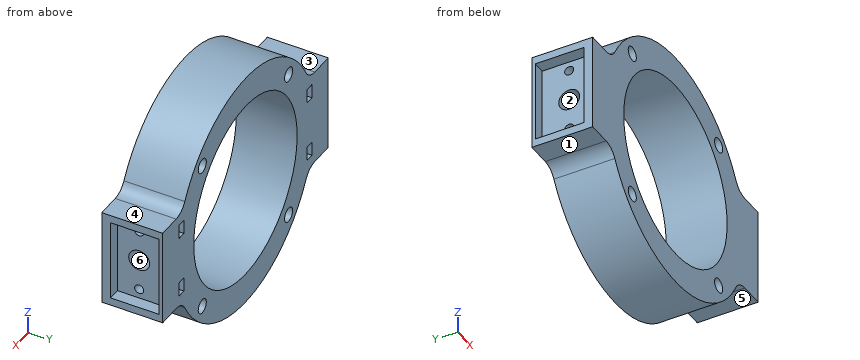
```python
from build123d import *

# Parameters (mm, degrees)
IZIM1_R                     = 52.5
Y_KSEKLIK_EKSTR_ZYON1_DEPTH = 35
IZIM2_R                     = 6.01
KES_EKSTR_ZYON1_DEPTH       = 27.24
IZIM3_W                     = 47
IZIM3_H                     = 28
KES_EKSTR_ZYON2_DEPTH       = 7
IZIM4_R                     = 2.6
KES_EKSTR_ZYON3_DEPTH       = 20
KES_EKSTR_ZYON4_DEPTH       = 2.45
IZIM7_R                     = 4.1
KES_EKSTR_ZYON5_DEPTH       = 115.808536268
RADYUS1_R                   = 10


with BuildPart() as part:
    # Çizim1 → Yükseklik-Ekstrüzyon1 (new body)
    with BuildSketch(Plane(origin=(0, 0, 0), x_dir=(1, 0, 0), z_dir=(0, 1, 0))):
        with BuildLine():
            Line((-64.156059729, 28), (-84, 28))
            Line((-84, 28), (-84, -28))
            Line((-84, -28), (-64.156059729, -28))
            ThreePointArc((-64.156059729, -28), (0, -70), (64.156059729, -28))
            Line((64.156059729, -28), (84, -28))
            Line((84, -28), (84, 28))
            Line((84, 28), (64.156059729, 28))
            ThreePointArc((64.156059729, 28), (0, 70), (-64.156059729, 28))
        make_face()
        with Locations(Location((0, 0, 0), (0, 0, 270))):
            Circle(IZIM1_R, mode=Mode.SUBTRACT)
    extrude(amount=Y_KSEKLIK_EKSTR_ZYON1_DEPTH)

    # Çizim2 → Kes-Ekstrüzyon1 (cut)
    with BuildSketch(Plane(origin=(84, 0, 0), x_dir=(0, 0, -1), z_dir=(1, 0, 0))):
        with Locations((0, 17.5)):
            Circle(IZIM2_R)
    kes_ekstr_zyon1 = extrude(amount=-KES_EKSTR_ZYON1_DEPTH, mode=Mode.SUBTRACT)

    # Aynalama1: Kes-Ekstrüzyon1 across plane
    add(kes_ekstr_zyon1.mirror(Plane(origin=(0, 0, 0), x_dir=(0, 0, 1), z_dir=(1, 0, 0))), mode=Mode.SUBTRACT)

    # Çizim3 → Kes-Ekstrüzyon2 (cut)
    with BuildSketch(Plane(origin=(84, 0, 0), x_dir=(0, 0, -1), z_dir=(1, 0, 0))):
        with Locations((0, 19)):
            Rectangle(IZIM3_W, IZIM3_H)
    kes_ekstr_zyon2 = extrude(amount=-KES_EKSTR_ZYON2_DEPTH, mode=Mode.SUBTRACT)

    # Aynalama2: Kes-Ekstrüzyon2 across plane
    add(kes_ekstr_zyon2.mirror(Plane(origin=(0, 0, 0), x_dir=(0, 0, 1), z_dir=(1, 0, 0))), mode=Mode.SUBTRACT)

    # Çizim4 → Kes-Ekstrüzyon3 (cut)
    with BuildSketch(Plane(origin=(77, 0, 0), x_dir=(0, 0, -1), z_dir=(1, 0, 0))):
        with Locations((18, 17.5)):
            Circle(IZIM4_R)
        with Locations(Location((-18, 17.5, 0), (0, 0, 180))):
            Circle(IZIM4_R)
    kes_ekstr_zyon3 = extrude(amount=-KES_EKSTR_ZYON3_DEPTH, mode=Mode.SUBTRACT)

    # Aynalama3: Kes-Ekstrüzyon3 across plane
    add(kes_ekstr_zyon3.mirror(Plane(origin=(0, 0, 0), x_dir=(0, 0, 1), z_dir=(1, 0, 0))), mode=Mode.SUBTRACT)

    # Çizim6 → Kes-Ekstrüzyon4 (cut, symmetric)
    with BuildSketch(Plane.ZY.offset(65)):
        Polygon((-22.1, 35), (-13.9, 35), (-13.9, 15.132863896), (-18, 12.765727793), (-22.1, 15.132863896), align=None)
        Polygon((18, 12.765727793), (22.1, 15.132863896), (22.1, 35), (13.9, 35), (13.9, 15.132863896), align=None)
    kes_ekstr_zyon4 = extrude(amount=KES_EKSTR_ZYON4_DEPTH, both=True, mode=Mode.SUBTRACT)

    # Aynalama4: Kes-Ekstrüzyon4 across plane
    add(kes_ekstr_zyon4.mirror(Plane(origin=(0, 0, 0), x_dir=(0, 0, 1), z_dir=(1, 0, 0))), mode=Mode.SUBTRACT)

    # Çizim7 → Kes-Ekstrüzyon5 (cut, through all)
    with BuildSketch(Plane(origin=(0, 35, 0), x_dir=(1, 0, 0), z_dir=(0, 1, 0))):
        with Locations(Location((43.840620434, -43.840620434, 0), (0, 0, 270))):
            Circle(IZIM7_R)
        with Locations(Location((-43.840620434, -43.840620434, 0), (0, 0, 270))):
            Circle(IZIM7_R)
        with Locations(Location((-43.840620434, 43.840620434, 0), (0, 0, 270))):
            Circle(IZIM7_R)
        with Locations(Location((43.840620434, 43.840620434, 0), (0, 0, 270))):
            Circle(IZIM7_R)
    extrude(amount=-KES_EKSTR_ZYON5_DEPTH, mode=Mode.SUBTRACT)

    # Radyus1
    radyus1_edges = [part.edges().sort_by_distance(p)[0] for p in [
        (64.156059729, 17.5, -28),
        (64.156059729, 17.5, 28),
        (-64.156059729, 17.5, 28),
        (-64.156059729, 17.5, -28),
    ]]
    fillet(radyus1_edges, radius=RADYUS1_R)


solid = part.part
```
Input: part model. Units: mm. Frame: model coordinates. Face numbers are marked on the shaded views. A direction names the side the tool comes from. Round coordinates to 2 decimals unless told otherwise and drop trailing zeros. Order: outer loops, then holes, each group sorted by start corner. A loop starts at its lowest first (then second) coordinate and runs counter-clockwise, first axis right, second up. Notation, with made-up numbers: (-25, 89) - (-11, 89) arc R26 ccw to (-11, 114) - close; hole circle Ø2 at (60.25, 33.5). An arc over 180 degrees is marked (long way). Answer in a Markdown table with one row per item.
Item 1: Pin query (flat end, axial travel): pin 1 (10 mm diameter, centred on x = -57.5, y = 20, fed in from +Z); pin 2 (12 mm diameter, centred on y = 16, z = 39, fed in from -X); pin 3 (2.5 mm diameter, centred on y = 17, z = -18.5, fed in from +X). Return the tip coordinate at first contact, or that it passes through.
Model answer:
| item | result |
|---|---|
| pin 1 | stops at z = 46.3 |
| pin 2 | stops at x = -61.74 |
| pin 3 | stops at x = 57 |
Item 2: Line query: line 1 (Z direction, x = -68.75, y = 17.5); line 2 (Z direction, x = -66.5, y = 15); line 3 (X direction, y = 31, z = 42). Output: solid intervals per line, ascending.
Model answer:
| item | result |
|---|---|
| line 1 | z = -28.14 to -20.6, -15.4 to -6.01, 6.01 to 15.4, 20.6 to 28.14 |
| line 2 | z = -28.79 to -21.87, -14.13 to -5.47, 5.47 to 14.13, 21.87 to 28.79 |
| line 3 | x = -56 to -47.5, -40.18 to -31.5, 31.5 to 40.18, 47.5 to 56 |
Item 3: Section query C-C (y = 9.5). Return the cut outline in (x, z).
Model answer:
| item | result |
|---|---|
| outline | (-84, -28) - (-70.4, -28) arc R10 cw to (-61.6, -33.25) arc R70 ccw to (61.6, -33.25) arc R10 cw to (70.4, -28) - (84, -28) - (84, -23.5) - (77, -23.5) - (77, 23.5) - (84, 23.5) - (84, 28) - (70.4, 28) arc R10 cw to (61.6, 33.25) arc R70 ccw to (-61.6, 33.25) arc R10 cw to (-70.4, 28) - (-84, 28) - (-84, 23.5) - (-77, 23.5) - (-77, -23.5) - (-84, -23.5) - close; hole circle Ø105 at (0, 0); hole circle Ø8.2 at (-43.84, -43.84); hole circle Ø8.2 at (-43.84, 43.84); hole circle Ø8.2 at (43.84, -43.84); hole circle Ø8.2 at (43.84, 43.84) |
Item 4: Section query B-B (z = 0). Return the cut outline in (x, y).
Model answer:
| item | result |
|---|---|
| outline | (-84, 0) - (-52.5, 0) - (-52.5, 35) - (-84, 35) - (-84, 33) - (-77, 33) - (-77, 23.51) - (-56.76, 23.51) - (-56.76, 11.49) - (-77, 11.49) - (-77, 5) - (-84, 5) - close; (52.5, 0) - (84, 0) - (84, 5) - (77, 5) - (77, 11.49) - (56.76, 11.49) - (56.76, 23.51) - (77, 23.51) - (77, 33) - (84, 33) - (84, 35) - (52.5, 35) - close |
Item 5: Section query A-A (x = 0). Return the cut outline in (y, z), then the cut area to 4 significant figures.
Model answer:
| item | result |
|---|---|
| outline | (0, -70) - (35, -70) - (35, -52.5) - (0, -52.5) - close; (0, 52.5) - (35, 52.5) - (35, 70) - (0, 70) - close |
| area | 1,225 mm² |
Item 6: Reachability of the marked faces 4, 5 and 6 from +Z, -Z, +X, -X, +Y, -Y: full face, straight path, thin tool, end or side. Return the list, or none.
Model answer:
| item | result |
|---|---|
| face 4 | +Z, +X, +Y, -Y |
| face 5 | -Z, +X, +Y, -Y |
| face 6 | +X |
Item 7: Section query D-D (z = -31). Return the cut outline in (x, y).
Model answer:
| item | result |
|---|---|
| outline | (-63.26, 0) - (-42.37, 0) - (-42.37, 35) - (-63.26, 35) - close; (42.37, 0) - (63.26, 0) - (63.26, 35) - (42.37, 35) - close |
Item 8: Mould query, pull axis Z, two halves, no side actions, for the marked faces 1, 2 and 3. Classes: released by +Z, released by -Z, zero draft, split by the parting line, or undercut.
Model answer:
| item | result |
|---|---|
| face 1 | released by -Z |
| face 2 | undercut |
| face 3 | released by +Z |
